from build123d import *

# Parameters (mm, degrees)
BASE_FLANGE1_START     = -3.048
BASE_FLANGE1_OUTLINE_R = 3.55
BASE_FLANGE1_DEPTH     = 3.048
CHAMFER1_SIZE          = 5.5
CHAMFER1_SIZE2         = 9.526279442
FILLET5_R              = 3
JOG1_START             = -32.26085306
JOG1_DEPTH             = 22.133833772
JOG1_START_2           = -30.91085306
JOG1_2_DEPTH           = 1.375
JOG1_START_3           = -23.98585306
JOG1_3_DEPTH           = 1.375
JOG1_START_4           = -30.914437073
JOG1_4_DEPTH           = 8.307168025
JOG1_5_DEPTH           = 15.25
FILLET4_R              = 3
CUT_EXTRUDE3_DEPTH     = 78.680918765
BOSS_EXTRUDE1_DEPTH    = 3.048
CUT_EXTRUDE4_REACH     = 59.066
SKETCH15_R             = 0.5


with BuildPart() as part:
    # Base-Flange1: read off the stored shape, not the designer's step
    # Base-Flange1 outline → Base-Flange1 (new body)
    with BuildSketch(Plane(origin=(0, 0, 0), x_dir=(0, 0, -1), z_dir=(1, 0, 0)).offset(BASE_FLANGE1_START)):
        with BuildLine():
            Line((11.76085306, 2.855261469), (28.086146356, 19.180554765))
            ThreePointArc((28.086146356, 19.180554765), (30.176735706, 22.309342834), (30.91085306, 26))
            Line((30.91085306, 26), (30.91085306, 26.390637175))
            ThreePointArc((30.91085306, 26.390637175), (32.26085306, 30), (30.91085306, 33.609362825))
            Line((30.91085306, 33.609362825), (30.91085306, 48.531723164))
            Line((30.91085306, 48.531723164), (30.914437073, 54.658476217))
            Line((30.914437073, 54.658476217), (30.91085306, 55.218276836))
            Line((30.91085306, 55.218276836), (30.91085306, 69))
            Line((30.91085306, 69), (22.61085306, 69))
            Line((22.61085306, 69), (22.61085306, 55.218276836))
            Line((22.61085306, 55.218276836), (22.607269048, 54.658476217))
            Line((22.607269048, 54.658476217), (22.61085306, 48.531723164))
            Line((22.61085306, 48.531723164), (22.61085306, 33.609362825))
            ThreePointArc((22.61085306, 33.609362825), (21.26085306, 30), (22.61085306, 26.390637175))
            Line((22.61085306, 26.390637175), (22.61085306, 25.443234037))
            Line((22.61085306, 25.443234037), (5.891866776, 8.724247753))
            Line((5.891866776, 8.724247753), (11.76085306, 2.855261469))
        make_face()
        with Locations((26.76085306, 30)):
            Circle(BASE_FLANGE1_OUTLINE_R, mode=Mode.SUBTRACT)
        with BuildLine():
            ThreePointArc((23.98585306, 64.875), (26.76085306, 67.65), (29.53585306, 64.875))
            Line((29.53585306, 64.875), (29.53585306, 51.875))
            ThreePointArc((29.53585306, 51.875), (26.76085306, 49.1), (23.98585306, 51.875))
            Line((23.98585306, 51.875), (23.98585306, 64.875))
        make_face(mode=Mode.SUBTRACT)
    extrude(amount=BASE_FLANGE1_DEPTH)

    # Chamfer1
    chamfer1_edges = [part.edges().sort_by_distance(p)[0] for p in [
        (-1.524, 8.724247753, -5.891866776),
    ]]
    chamfer1_side = [part.faces().sort_by_distance(p)[0] for p in [
        (-1.524, 5.789754611, -8.826359918),
    ]]
    chamfer(chamfer1_edges, length=CHAMFER1_SIZE, length2=CHAMFER1_SIZE2, reference=chamfer1_side[0])

    # Fillet5
    fillet5_edges = [part.edges().sort_by_distance(p)[0] for p in [
        (-1.524, 15.460344546, -12.627963569),
        (-1.524, 4.835160456, -9.780954073),
    ]]
    fillet(fillet5_edges, radius=FILLET5_R)

    # Jog1: read off the stored shape, not the designer's step
    # Jog1 outline → Jog1 (cut)
    with BuildSketch(Plane.XY.offset(JOG1_START)):
        with BuildLine():
            ThreePointArc((-3.048, 35.406615264), (-2.231290862, 38.454615264), (0, 40.685906126))
            Line((0, 40.685906126), (0, 69))
            Line((0, 69), (-3.048, 69))
            Line((-3.048, 69), (-3.048, 35.406615264))
        make_face()
    extrude(amount=JOG1_DEPTH, mode=Mode.SUBTRACT)

    # Jog1 2 outline → Jog1 2 (add)
    with BuildSketch(Plane.XY.offset(JOG1_START_2)):
        with BuildLine():
            ThreePointArc((0, 35.406615264), (0.477342873, 37.04430447), (1.759859538, 38.169041399))
            Line((1.759859538, 38.169041399), (11.730280924, 42.818325246))
            ThreePointArc((11.730280924, 42.818325246), (14.295314254, 45.067799104), (15.25, 48.343177516))
            Line((15.25, 48.343177516), (15.25, 69))
            Line((15.25, 69), (12.202, 69))
            Line((12.202, 69), (12.202, 48.343177516))
            ThreePointArc((12.202, 48.343177516), (11.724657127, 46.70548831), (10.442140462, 45.580751381))
            Line((10.442140462, 45.580751381), (0.471719076, 40.931467534))
            ThreePointArc((0.471719076, 40.931467534), (0.233180454, 40.813833303), (0, 40.685906126))
            Line((0, 40.685906126), (0, 35.406615264))
        make_face()
    extrude(amount=JOG1_2_DEPTH)

    # Jog1 3 outline → Jog1 3 (add)
    with BuildSketch(Plane.XY.offset(JOG1_START_3)):
        with BuildLine():
            ThreePointArc((0, 35.406615264), (0.477342873, 37.04430447), (1.759859538, 38.169041399))
            Line((1.759859538, 38.169041399), (11.730280924, 42.818325246))
            ThreePointArc((11.730280924, 42.818325246), (14.295314254, 45.067799104), (15.25, 48.343177516))
            Line((15.25, 48.343177516), (15.25, 69))
            Line((15.25, 69), (12.202, 69))
            Line((12.202, 69), (12.202, 48.343177516))
            ThreePointArc((12.202, 48.343177516), (11.724657127, 46.70548831), (10.442140462, 45.580751381))
            Line((10.442140462, 45.580751381), (0.471719076, 40.931467534))
            ThreePointArc((0.471719076, 40.931467534), (0.233180454, 40.813833303), (0, 40.685906126))
            Line((0, 40.685906126), (0, 35.406615264))
        make_face()
    extrude(amount=JOG1_3_DEPTH)

    # Jog1 4 outline → Jog1 4 (add)
    with BuildSketch(Plane.XY.offset(JOG1_START_4)):
        with BuildLine():
            ThreePointArc((0, 35.406615264), (0.477342873, 37.04430447), (1.759859538, 38.169041399))
            Line((1.759859538, 38.169041399), (11.730280924, 42.818325246))
            ThreePointArc((11.730280924, 42.818325246), (14.295314254, 45.067799104), (15.25, 48.343177516))
            Line((15.25, 48.343177516), (15.25, 69))
            Line((15.25, 69), (12.202, 69))
            Line((12.202, 69), (12.202, 48.343177516))
            ThreePointArc((12.202, 48.343177516), (11.724657127, 46.70548831), (10.442140462, 45.580751381))
            Line((10.442140462, 45.580751381), (0.471719076, 40.931467534))
            ThreePointArc((0.471719076, 40.931467534), (0.233180454, 40.813833303), (0, 40.685906126))
            Line((0, 40.685906126), (0, 35.406615264))
        make_face()
    extrude(amount=JOG1_4_DEPTH)

    # Jog1 5 outline → Jog1 5 (cut)
    with BuildSketch(Plane.YZ):
        Polygon((48.531723164, -30.91085306), (34, -30.91085306), (34, -30.914437073), (54.658476217, -30.914437073), align=None)
        Polygon((34, -22.607269048), (34, -22.61085306), (48.531723164, -22.61085306), (54.658476217, -22.607269048), align=None)
        Polygon((55.218276836, -30.91085306), (54.658476217, -30.914437073), (70, -30.914437073), (70, -30.91085306), align=None)
        Polygon((70, -22.607269048), (54.658476217, -22.607269048), (55.218276836, -22.61085306), (70, -22.61085306), align=None)
        with BuildLine():
            Line((64.875, -23.98585306), (51.875, -23.98585306))
            ThreePointArc((51.875, -23.98585306), (49.1, -26.76085306), (51.875, -29.53585306))
            Line((51.875, -29.53585306), (64.875, -29.53585306))
            ThreePointArc((64.875, -29.53585306), (67.65, -26.76085306), (64.875, -23.98585306))
        make_face()
    extrude(amount=JOG1_5_DEPTH, mode=Mode.SUBTRACT)

    # Fillet4
    fillet4_edges = [part.edges().sort_by_distance(p)[0] for p in [
        (13.726, 69, -30.91085306),
        (13.726, 69, -22.61085306),
    ]]
    fillet(fillet4_edges, radius=FILLET4_R)

    # Sketch14<4> → Cut-Extrude3 (cut, through all)
    with BuildSketch(Plane(origin=(0, 0, 0), x_dir=(0, 0, -1), z_dir=(1, 0, 0))):
        Polygon((11.500086567, 5.024730268), (12.821513232, 3.915921641), (25.065698027, 16.160106436), (22.588172835, 18.238996911), align=None)
        Polygon((25.065698027, 16.160106436), (12.821513232, 3.915921641), (14.142939896, 2.807113014), (25.231026163, 16.021379658), align=None)
    extrude(amount=-CUT_EXTRUDE3_DEPTH, mode=Mode.SUBTRACT)

    # Sketch14 → Boss-Extrude1 (add)
    with BuildSketch(Plane(origin=(0, 0, 0), x_dir=(0, 0, -1), z_dir=(1, 0, 0))):
        with BuildLine():
            Line((12.821513232, 3.915921641), (11.76085306, 2.855261469))
            Line((11.76085306, 2.855261469), (12.761421716, 1.854692814))
            ThreePointArc((12.761421716, 1.854692814), (14.450555595, 1.197824573), (16.07601197, 1.999410949))
            Line((16.07601197, 1.999410949), (26.76311505, 14.735804439))
            ThreePointArc((26.76311505, 14.735804439), (26.992415169, 15.474972553), (26.625555608, 16.156413752))
            ThreePointArc((26.625555608, 16.156413752), (26.255439336, 16.881363004), (26.546933828, 17.641342237))
            Line((26.546933828, 17.641342237), (25.065698027, 16.160106436))
            Line((25.065698027, 16.160106436), (25.231026163, 16.021379658))
            Line((25.231026163, 16.021379658), (14.142939896, 2.807113014))
            Line((14.142939896, 2.807113014), (12.821513232, 3.915921641))
        make_face()
    extrude(amount=-BOSS_EXTRUDE1_DEPTH)

    # Sketch15 → Cut-Extrude4 (cut, up to next)
    with BuildSketch(Plane(origin=(-15.593409677, 33.440174967, 0), x_dir=(0.906307787036651, 0.4226182617406973, 0), z_dir=(-0.4226182617406973, 0.906307787036651, 0)), mode=Mode.PRIVATE) as cut_extrude4_sk1:
        with Locations(Location((23.226479732, 26.76085306, 0), (0, 0, 180))):
            Circle(SKETCH15_R)
    cut_extrude4_tool1 = extrude(cut_extrude4_sk1.sketch, amount=-CUT_EXTRUDE4_REACH, mode=Mode.PRIVATE) & part.part
    add(cut_extrude4_tool1.solids().sort_by_distance((5.45693, 43.256109, -26.760853))[0], mode=Mode.SUBTRACT)


solid = part.part
Part model, mm, in its own coordinate system. A direction names the side the tool comes from. Coordinates: 2 decimals unless noted, no trailing zeros. Write each loop counter-clockwise with the first axis right and the second up, starting at its lowest first coordinate (ties: lowest second). Pieces come first, ordered by that corner, then holes. Notation, with made-up numbers: M 6,17.25 L 13,17.25 A18 cw 13,22.25 Z; hole C -36.75,-39 d11. An arc over 180 degrees is marked long. Return JSON: item names as keys, results as strings.
1. 3-axis set-ups, long thin cutter, end or side, ignore diameter. For faces 4 (the face through (-1.545, 18.4, -27.306)), 5 (the face through (0, 20, -21)), 6 (the face through (14, 58, -29.536)), 7 (the face through (6.151, 41.922, -26.265)): which of +Z, -Z, +X, -X, +Y, -Y reach the whole face in a straight line?
Determined:
{"face 4": "-Z, +X, -X", "face 5": "+Z, -Z, +X, -Y", "face 6": "+X, -X", "face 7": "none"}
2. Saw through at A-A, the plane y = 30. Write the cut outline in (x, z).
Determined:
{"outline": "M -3.05,-32.26 L 0,-32.26 L 0,-30.31 L -3.05,-30.31 Z; M -3.05,-23.21 L 0,-23.21 L 0,-21.26 L -3.05,-21.26 Z"}
3. Probe L1, parallel to X at y = 34, z = -29; L2, parallel to Y at x = -0.25, z = -16.25; L3, parallel to Z at x = 6.25, y = 41. List the from-to ranges inside material, lowest first.
Determined:
{"L1": "-3.05 to 0", "L2": "2.21 to 5.32, 10.69 to 19.08", "L3": "-30.91 to -27.2, -26.32 to -22.61"}
4. Saw through at B-B, the plane y = 12. Write the cut outline in (x, z), then the cut area to 3 significant figures.
Determined:
{"outline": "M -3.05,-24.47 L 0,-24.47 L 0,-21.86 L -3.05,-21.86 Z; M -3.05,-17.35 L 0,-17.35 L 0,-11.7 L -3.05,-11.7 Z", "area": "25.2 mm²"}
5. Pull direction Z, two halves, no side cores. Call faces 1 (the face through (-1.5, 11.7, -17.1)), 2 (the face through (-1.55, 10.65, -11.34)), 3 (the face through (14.27, 45.03, -26.82)): pulls with the +Z half, pulls with the -Z half, needs draft (parallel to the pull), parting line crosses it, or undercut.
Determined:
{"face 1": "undercut", "face 2": "pulls with the +Z half", "face 3": "needs draft"}
6. Flat gauge pins, fed straight in: pin 1 Ø1 at (x, y) = (6.5, 44) entering from -Z; pin 2 Ø3 at (x, z) = (9.5, -22.5) entering from -Y; pin 3 Ø8 at (y, z) = (30, -26.76) entering from +X. Where does each tip first touch, or does it go through?
Determined:
{"pin 1": "z = -30.91", "pin 2": "y = 41.08", "pin 3": "x = 0"}
7. Saw through at C-C, the plane y = 47. Write the cut outline in (x, z), then the cut area to 3 significant figures.
Determined:
{"outline": "M 11.89,-30.91 L 15.1,-30.91 L 15.1,-22.61 L 11.89,-22.61 Z", "area": "26.6 mm²"}
